For this review, take the finished solid that the model builds, in its own axes (mm). Face numbers are marked on the shaded views. A direction names the side the tool comes from. Coordinates: 2 decimals unless noted, no trailing zeros. Loops run counter-clockwise (first coordinate to the right, second up) from the corner with the lowest first, then second, coordinate; pieces in that order, holes last. Notation, with made-up numbers: M 31,-16 L 58,-16 A24 cw 58,2 Z; hole C 68,87.25 d7. An arc over 180 degrees is marked long. Write item = value, one per line.
from build123d import *

# Parameters (mm, degrees)
SKETCH1_R           = 60.5
SKETCH1_R_2         = 50.5
SKETCH1_R_3         = 42.5
BOSS_EXTRUDE1_DEPTH = 15
SKETCH2_R           = 7.5
CUT_EXTRUDE1_DEPTH  = 7
SKETCH3_R           = 3.15
CUT_EXTRUDE2_DEPTH  = 15
FILLET1_R           = 4
SKETCH4_R           = 10
BOSS_EXTRUDE2_DEPTH = 8
CHAMFER1_SIZE       = 1


with BuildPart() as part:
    # Sketch1 → Boss-Extrude1 (new body)
    # profile 1 of 4: a face of its own
    with BuildSketch(Plane(origin=(0, 0, 0), x_dir=(1, 0, 0), z_dir=(0, 1, 0))):
        with Locations(Location((0, 0, 0), (0, 0, 270))):
            Circle(SKETCH1_R)
        Circle(SKETCH1_R_2, mode=Mode.SUBTRACT)
    # profile 2 of 4: a face of its own
    with BuildSketch(Plane(origin=(0, 0, 0), x_dir=(1, 0, 0), z_dir=(0, 1, 0))):
        with BuildLine():
            ThreePointArc((-27.318473412, 32.556888833), (0, 42.5), (27.318473412, 32.556888833))
            Line((27.318473412, 32.556888833), (32.460774289, 38.685244378))
            ThreePointArc((32.460774289, 38.685244378), (0, 50.5), (-32.460774289, 38.685244378))
            Line((-32.460774289, 38.685244378), (-27.318473412, 32.556888833))
        make_face()
    # profile 3 of 4: a face of its own
    with BuildSketch(Plane(origin=(0, 0, 0), x_dir=(1, 0, 0), z_dir=(0, 1, 0))):
        Circle(SKETCH1_R_3)
    # profile 4 of 4: a face of its own
    with BuildSketch(Plane(origin=(0, 0, 0), x_dir=(1, 0, 0), z_dir=(0, 1, 0))):
        with BuildLine():
            Line((32.460774289, -38.685244378), (27.318473412, -32.556888833))
            ThreePointArc((27.318473412, -32.556888833), (0, -42.5), (-27.318473412, -32.556888833))
            Line((-27.318473412, -32.556888833), (-32.460774289, -38.685244378))
            ThreePointArc((-32.460774289, -38.685244378), (0, -50.5), (32.460774289, -38.685244378))
        make_face()
    extrude(amount=BOSS_EXTRUDE1_DEPTH)

    # Sketch2 → Cut-Extrude1 (cut)
    with BuildSketch(Plane(origin=(0, 15, 0), x_dir=(1, 0, 0), z_dir=(0, 1, 0))):
        with Locations(Location((-27, 0, 0), (0, 0, 270))):
            Circle(SKETCH2_R)
        with Locations(Location((27, 0, 0), (0, 0, 270))):
            Circle(SKETCH2_R)
    extrude(amount=-CUT_EXTRUDE1_DEPTH, mode=Mode.SUBTRACT)

    # Sketch3 → Cut-Extrude2 (cut)
    with BuildSketch(Plane(origin=(0, 15, 0), x_dir=(1, 0, 0), z_dir=(0, 1, 0))):
        with Locations(Location((-27, 0, 0), (0, 0, 270))):
            Circle(SKETCH3_R)
        with Locations(Location((27, 0, 0), (0, 0, 270))):
            Circle(SKETCH3_R)
    extrude(amount=-CUT_EXTRUDE2_DEPTH, mode=Mode.SUBTRACT)

    # Fillet1
    fillet1_edges = [part.edges().sort_by_distance(p)[0] for p in [
        (32.460774289, 7.5, 38.685244378),
        (27.318473412, 7.5, 32.556888833),
        (-27.318473412, 7.5, 32.556888833),
        (-32.460774289, 7.5, 38.685244378),
        (32.460774289, 7.5, -38.685244378),
        (27.318473412, 7.5, -32.556888833),
        (-27.318473412, 7.5, -32.556888833),
        (-32.460774289, 7.5, -38.685244378),
    ]]
    fillet(fillet1_edges, radius=FILLET1_R - 0.0001)  # a hair under: the kernel refuses the full size

    # Sketch4 → Boss-Extrude2 (add)
    with BuildSketch(Plane(origin=(0, 15, 0), x_dir=(1, 0, 0), z_dir=(0, 1, 0))):
        with Locations(Location((0, 0, 0), (0, 0, 270))):
            Circle(SKETCH4_R)
    extrude(amount=BOSS_EXTRUDE2_DEPTH)

    # Chamfer1
    chamfer1_edges = [part.edges().sort_by_distance(p)[0] for p in [
        (0, 23, -10),
    ]]
    chamfer(chamfer1_edges, length=CHAMFER1_SIZE)


solid = part.part
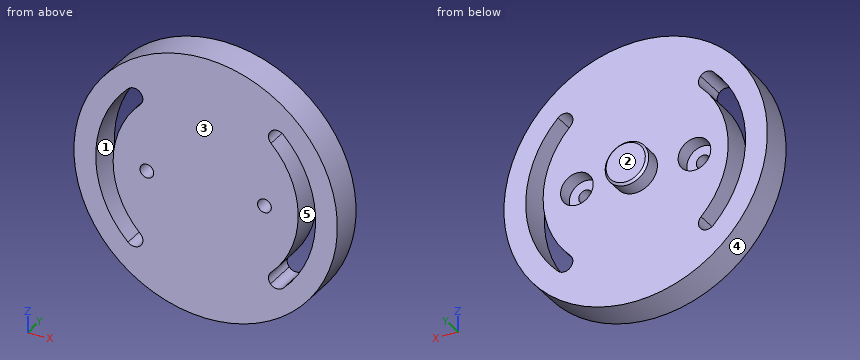
Q1. Machinability: for the marked faces 1 and 2, which of the approach directions +Z, -Z, +X, -X, +Y, -Y give a long, thin tool a straight path to every point of the face, cutting with its end or side? Answer none if there is none.
Solved:
face_1 = +Y, -Y
face_2 = +Z, -Z, +X, -X, +Y
Q2. For pin 1 Ø17 at (x, z) = (-27, 0) entering from +Y; pin 2 Ø6 at (x, y) = (-14, 17.5) entering from +Z; pin 3 Ø7.5 at (x, z) = (-25, -0.5) entering from +Y, all flat-tipped, find the tip position at first contact; note any pin that passes through.
Solved:
pin_1 = 15
pin_2 = 59.23
pin_3 = 8
Q3. Add section C-C (z = 18). Write out the cut boundary in (x, y).
Solved:
outline = M -57.76,0 L -47.18,0 L -47.18,15 L -57.76,15 Z; M -38.5,0 L 38.5,0 L 38.5,15 L -38.5,15 Z; M 47.18,0 L 57.76,0 L 57.76,15 L 47.18,15 Z
Q4. Draft analysis for pull direction Z (two halves, no side actions). For the marked faces 3, 4 and 5, state which applies: +Z half, -Z half, draft (parallel to the pull), parting line (faces both ways), or undercut.
Solved:
face_3 = draft
face_4 = parting line
face_5 = undercut
Q5. For line 1 along X through (y, z) = (6.5, 0); line 2 along X through (y, z) = (13.75, 0); line 3 along X through (y, z) = (12.25, 15), list the stretches that pass through material, from the lowest coordinate up.
Solved:
line_1 = -60.5 to -50.5, -42.5 to -30.15, -23.85 to 23.85, 30.15 to 42.5, 50.5 to 60.5
line_2 = -60.5 to -50.5, -42.5 to -34.5, -19.5 to 19.5, 34.5 to 42.5, 50.5 to 60.5
line_3 = -58.61 to -48.22, -39.76 to 39.76, 48.22 to 58.61
Q6. Add section A-A (y = 4.5). State how many separate pieces and enclosed holes the cut face has, and give its area (3 significant figures).
Solved:
separate_pieces = 1
enclosed_holes = 4
area = 10,200 mm²
Q7. Add section D-D (x = -27). Write out the cut boundary in (y, z), and give its area (3 significant figures).
Solved:
outline = M 0,-54.14 L 15,-54.14 L 15,-7.5 L 8,-7.5 L 8,-3.15 L 0,-3.15 Z; M 0,3.15 L 8,3.15 L 8,7.5 L 15,7.5 L 15,54.14 L 0,54.14 Z
area = 1,470 mm²
